Geometry check sheet. Reference: the model listing, model coordinates, mm. Give positions to 0.01 mm unless a question says otherwise; leave off trailing zeros. Write each loop counter-clockwise with the first axis right and the second up, starting at its lowest first coordinate (ties: lowest second). Pieces come first, ordered by that corner, then holes. Notation, with made-up numbers: (34.25, -1) -> (89.25, -1) arc R18 ccw to (89.25, 27) -> close; hole circle Ø4 at (-36.75, 55.25). An arc over 180 degrees is marked (long way). Use a Markdown table: item, result. Add a question column.
from build123d import *

# Parameters (mm, degrees)
F1_DEPTH = 5
F2_R     = 5
F3_DEPTH = 25


with BuildPart() as f1:
    # F0 (on Front) → F1 (new body)
    with BuildSketch(Plane.XZ):
        with BuildLine():
            ThreePointArc((-10, 80), (0, 70), (10, 80))
            ThreePointArc((10, 80), (0, 90), (-10, 80))
        make_face()
        with BuildLine():
            Line((10, -80), (10, 80))
            ThreePointArc((10, 80), (0, 70), (-10, 80))
            Line((-10, 80), (-10, -80))
            ThreePointArc((-10, -80), (0, -70), (10, -80))
        make_face()
        with BuildLine():
            ThreePointArc((-10, -80), (0, -90), (10, -80))
            ThreePointArc((10, -80), (0, -70), (-10, -80))
        make_face()
    extrude(amount=F1_DEPTH)

    # F2 (on face) → F3 (cut)
    with BuildSketch(Plane.XZ.offset(5)):
        with Locations((0, 80)):
            Circle(F2_R)
        with Locations((0, -80)):
            Circle(F2_R)
        Circle(F2_R)
    extrude(amount=-F3_DEPTH, mode=Mode.SUBTRACT)


solid = f1.part
1) Draft check along X on faces 1 (the face through (10, -2, -1)), 2 (the face through (-10, -2, 1)), 3 (the face through (-1.08, -2.54, -84.88)). Enter one of: +X half, -X half, draft (parallel to the pull), parting line (faces both ways), or undercut.
2) Gauge pin test, flat end, axial feed: P1, Ø9, axis at x = 0, z = 0, coming from the -Y side. Record the tip position at first contact, or that the pin passes through.
3) Sectioned sample at C-C, the plane y = -4.05. Enter the section's corners in (x, z).
4) Material ranges on probe 1 along Z at (x, y) = (0, -2.8); probe 2 along Z at (x, y) = (0.75, -4.2); probe 3 along X at (y, z) = (-2.4, -79.5), recorded low to high. Write a range as [from, to].
5) Sectioned sample at A-A, the plane z = 0. Enter the section's corners in (x, y), and give its area (3 significant figures).
6) Sectioned sample at D-D, the plane x = 7.25. Enter the section's corners in (y, z), and give its area (3 significant figures).
7) Sectioned sample at B-B, the plane x = 0. Enter the section's corners in (y, z), and give its area (3 significant figures).
Check values:
| question | item | result |
|---|---|---|
| 1 | face 1 | +X half |
| 1 | face 2 | -X half |
| 1 | face 3 | undercut |
| 2 | P1 | through |
| 3 | outline | (-10, -80) arc R10 ccw to (10, -80) -> (10, 80) arc R10 ccw to (-10, 80) -> close; hole circle Ø10 at (0, -80); hole circle Ø10 at (0, 0); hole circle Ø10 at (0, 80) |
| 4 | probe 1 | [-90, -85], [-75, -5], [5, 75], [85, 90] |
| 4 | probe 2 | [-89.97, -84.94], [-75.06, -4.94], [4.94, 75.06], [84.94, 89.97] |
| 4 | probe 3 | [-10, -4.97], [4.97, 10] |
| 5 | outline | (-10, -5) -> (-5, -5) -> (-5, 0) -> (-10, 0) -> close; (5, -5) -> (10, -5) -> (10, 0) -> (5, 0) -> close |
| 5 | area | 50.0 mm² |
| 6 | outline | (-5, -86.89) -> (0, -86.89) -> (0, 86.89) -> (-5, 86.89) -> close |
| 6 | area | 869 mm² |
| 7 | outline | (-5, -90) -> (0, -90) -> (0, -85) -> (-5, -85) -> close; (-5, -75) -> (0, -75) -> (0, -5) -> (-5, -5) -> close; (-5, 5) -> (0, 5) -> (0, 75) -> (-5, 75) -> close; (-5, 85) -> (0, 85) -> (0, 90) -> (-5, 90) -> close |
| 7 | area | 750 mm² |
